from build123d import *

# Parameters (mm, degrees)
F1_DEPTH       = 25.4
F2_R           = 6.35
F3_DEPTH       = 25.4
F4_R           = 5.08
F5_R           = 2.54
F7_D           = 5.1054
F7_DEPTH       = 25.4
F7_CSINK_D     = 5.588
F7_CSINK_ANGLE = 82
F7_TIP         = 1.5338169022


with BuildPart() as f1:
    # F0 (on Top) → F1 (new body)
    with BuildSketch(Plane.XY):
        Polygon((0, 50.8), (0, 0), (-50.8, 0), (-50.8, -38.1), (38.1, -38.1), (38.1, 50.8), align=None)
    extrude(amount=F1_DEPTH)

    # F2 (on face) → F3 (cut, through all)
    with BuildSketch(Plane.XY.offset(25.4)):
        with Locations((-31.75, -19.05)):
            Circle(F2_R)
    extrude(amount=-F3_DEPTH, mode=Mode.SUBTRACT)

    # F4
    f4_edges = [f1.edges().sort_by_distance(p)[0] for p in [
        (-50.8, -38.1, 12.7),
        (-50.8, 0, 12.7),
        (0, 0, 12.7),
        (0, 50.8, 12.7),
    ]]
    fillet(f4_edges, radius=F4_R)

    # F5
    f5_edges = [f1.edges().sort_by_distance(p)[0] for p in [
        (-3.81, -38.1, 25.4),
    ]]
    fillet(f5_edges, radius=F5_R)

    # F7
    with Locations(Plane.YZ.offset(38.1)):
        with Locations((29.21, 12.7), (-16.51, 12.7)):
            CounterSinkHole(F7_D / 2, F7_CSINK_D / 2, depth=F7_DEPTH, counter_sink_angle=F7_CSINK_ANGLE)
            with Locations((0, 0, -(F7_DEPTH + F7_TIP / 2))):  # 118° drill point
                Cone(0, F7_D / 2, F7_TIP, mode=Mode.SUBTRACT)


solid = f1.part
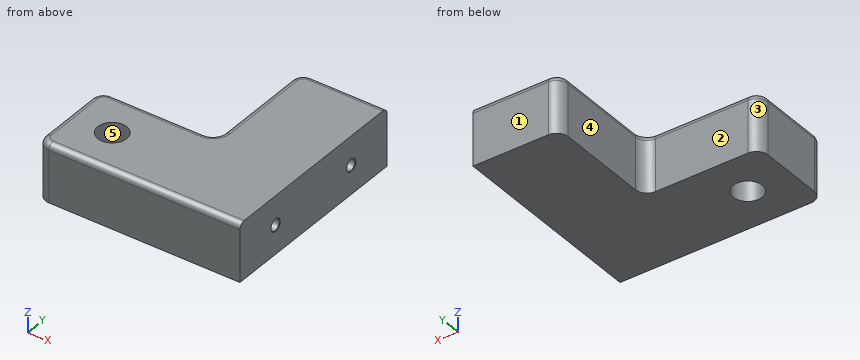
Geometry check sheet. Reference: the model listing, model coordinates, mm. Face numbers are marked on the shaded views. A direction names the side the tool comes from. Give positions to 0.01 mm unless a question says otherwise; leave off trailing zeros. Order: outer loops, then holes, each group sorted by start corner. A loop starts at its lowest first (then second) coordinate and runs counter-clockwise, first axis right, second up. Notation, with made-up numbers: (-33.75, -17.5) - (-29.75, -17.5) arc R30 cw to (-29.75, 17.5) - close; hole circle Ø1 at (85.5, 0). An arc over 180 degrees is marked (long way). Answer as a JSON object with one key per item and string values.
(1) Cross-section at C-C (z = 17). Record the cut outline in (x, y), then the cut area to 3 significant figures.
Report:
{"outline": "(-50.8, -33.02) arc R5.08 ccw to (-45.72, -38.1) - (38.1, -38.1) - (38.1, 50.8) - (5.08, 50.8) arc R5.08 ccw to (0, 45.72) - (0, 5.08) arc R5.08 cw to (-5.08, 0) - (-45.72, 0) arc R5.08 ccw to (-50.8, -5.08) - close; hole circle Ø12.7 at (-31.75, -19.05)", "area": "5,180 mm^2"}
(2) Cross-section at D-D (y = 19). Record the cut outline in (x, z), then the cut area to 3 significant figures.
Report:
{"outline": "(0, 0) - (38.1, 0) - (38.1, 25.4) - (2.54, 25.4) arc R2.54 ccw to (0, 22.86) - close", "area": "966 mm^2"}
(3) Cross-section at A-A (x = -31.75). Record the cut outline in (y, z).
Report:
{"outline": "(-38.1, 0) - (-25.4, 0) - (-25.4, 25.4) - (-35.56, 25.4) arc R2.54 ccw to (-38.1, 22.86) - close; (-12.7, 0) - (0, 0) - (0, 22.86) arc R2.54 ccw to (-2.54, 25.4) - (-12.7, 25.4) - close"}
(4) Depth check by flat-ended pin: pin 1 Ø2 at (x, z) = (2, 11) entering from +Y; pin 2 Ø4 at (y, z) = (29.21, 12.7) entering from +X; pin 3 Ø8 at (x, z) = (-11.5, 19.5) entering from +Y. Enter the tip coordinate at first touch or a pass-through.
Report:
{"pin 1": "y = 50.35", "pin 2": "x = 12.37", "pin 3": "y = 0"}
(5) Tool access check on the marked faces 1 and 2. Record the directions out of +Z, -Z, +X, -X, +Y, -Y that give a thin tool (end or side, any length) a straight path to the whole face; none if there is none.
Report:
{"face 1": "+Z, -Z, +X, -X, +Y", "face 2": "+Z, -Z, -X, +Y"}
(6) Draft check along Y on the marked faces 3, 4 and 5. Enter one of: released by +Y, released by -Y, zero draft, split by the parting line, or undercut.
Report:
{"face 3": "released by +Y", "face 4": "zero draft", "face 5": "undercut"}
(7) Material ranges on line 1 (Y direction, x = 23.25, z = 12.7); line 2 (Y direction, x = -31.75, z = 11.5); line 3 (Y direction, x = -6.5, z = 1.5), recorded low to high.
Report:
{"line 1": "-38.1 to -19.06, -13.96 to 26.66, 31.76 to 50.8", "line 2": "-38.1 to -25.4, -12.7 to 0", "line 3": "-38.1 to 0"}
(8) Cross-section at B-B (x = 25.5). Record the cut outline in (y, z).
Report:
{"outline": "(-38.1, 0) - (50.8, 0) - (50.8, 22.86) arc R2.54 ccw to (48.26, 25.4) - (-35.56, 25.4) arc R2.54 ccw to (-38.1, 22.86) - close; hole circle Ø5.11 at (-16.51, 12.7); hole circle Ø5.11 at (29.21, 12.7)"}
